```python
from build123d import *

# Parameters (mm, degrees)
SKETCH1_R           = 3.5
SKETCH1_R_2         = 1.5
BOSS_EXTRUDE1_DEPTH = 3
SKETCH2_R           = 3
SKETCH2_R_2         = 2
CUT_EXTRUDE1_DEPTH  = 0.3
CUT_EXTRUDE2_START  = -3
SKETCH2_2_R         = 3
SKETCH2_2_R_2       = 2
CUT_EXTRUDE2_DEPTH  = 0.3


with BuildPart() as part:
    # Sketch1 → Boss-Extrude1 (new body)
    with BuildSketch(Plane.XY):
        Circle(SKETCH1_R)
        Circle(SKETCH1_R_2, mode=Mode.SUBTRACT)
    extrude(amount=BOSS_EXTRUDE1_DEPTH)

    # Sketch2 → Cut-Extrude1 (cut)
    with BuildSketch(Plane.XY.offset(3)):
        Circle(SKETCH2_R)
        Circle(SKETCH2_R_2, mode=Mode.SUBTRACT)
    extrude(amount=-CUT_EXTRUDE1_DEPTH, mode=Mode.SUBTRACT)

    # Sketch2<2> → Cut-Extrude2 (cut)
    with BuildSketch(Plane.XY.offset(3).offset(CUT_EXTRUDE2_START)):
        Circle(SKETCH2_2_R)
        Circle(SKETCH2_2_R_2, mode=Mode.SUBTRACT)
    extrude(amount=CUT_EXTRUDE2_DEPTH, mode=Mode.SUBTRACT)


solid = part.part
```
The listing builds one solid part. Answer for the finished solid, in the listing's coordinates (mm). A direction names the side the tool comes from. Give positions to 0.01 mm unless a question says otherwise; leave off trailing zeros. Order: outer loops, then holes, each group sorted by start corner. A loop starts at its lowest first (then second) coordinate and runs counter-clockwise, first axis right, second up. Notation, with made-up numbers: M 83.5,63.25 L 92.5,63.25 A30 ccw 92.5,102.25 Z; hole C 1,48 d5. An arc over 180 degrees is marked long. Put each result on its own line as item: value. Start each with the question number.
Item 1: The part is cut by section C-C, the plane y = -2.25. Determine the outline of the cut face in (x, z).
Item 2: The part is cut by section D-D, the plane z = 0.6. Determine the outline of the cut face in (x, y).
Item 3: For a pull along X with two mould halves and no side action, classify faces 4 (the face through (3.233, -1.341, 1.479)), 5 (the face through (3, 1, 3)), 6 (the face through (-1.5, 0.07, 1.48)) as +X half, -X half, draft (parallel to the pull), parting line (faces both ways), or undercut.
Item 4: Which of the six approach directions +Z, -Z, +X, -X, +Y, -Y give full straight-line access (tool end or side, diameter ignored) to faces 1 (the face through (1, -2, 0.3)), 2 (the face through (1, -2, 2.7)), 3 (the face through (3, 1, 0))?
Item 5: The part is cut by section A-A, the plane y = 0. Determine the outline of the cut face in (x, z).
Item 6: Find the intervals of material crossed by line 1 along Y through (x, z) = (0, 0.15); line 2 along Y through (x, z) = (0, 1.25); line 3 along Z through (x, y) = (2.75, -0.25), in increasing order.
Answer key:
1. outline: M -2.68,0 L -1.98,0 L -1.98,0.3 L 1.98,0.3 L 1.98,0 L 2.68,0 L 2.68,3 L 1.98,3 L 1.98,2.7 L -1.98,2.7 L -1.98,3 L -2.68,3 Z
2. outline: C 0,0 d7; hole C 0,0 d3
3. face 4: parting line
3. face 5: draft
3. face 6: undercut
4. face 1: -Z
4. face 2: +Z
4. face 3: -Z, +X, -X, +Y, -Y
5. outline: M -3.5,0 L -3,0 L -3,0.3 L -2,0.3 L -2,0 L -1.5,0 L -1.5,3 L -2,3 L -2,2.7 L -3,2.7 L -3,3 L -3.5,3 Z; M 1.5,0 L 2,0 L 2,0.3 L 3,0.3 L 3,0 L 3.5,0 L 3.5,3 L 3,3 L 3,2.7 L 2,2.7 L 2,3 L 1.5,3 Z
6. line 1: y = -3.5 to -3, -2 to -1.5, 1.5 to 2, 3 to 3.5
6. line 2: y = -3.5 to -1.5, 1.5 to 3.5
6. line 3: z = 0.3 to 2.7
